Geometry check sheet. Reference: the model listing, model coordinates, mm. A direction names the side the tool comes from. Round coordinates to 2 decimals unless told otherwise and drop trailing zeros. Loops run counter-clockwise (first coordinate to the right, second up) from the corner with the lowest first, then second, coordinate; pieces in that order, holes last.
```python
from build123d import *

# Parameters (mm, degrees)
SKETCH1_R           = 6.35
BOSS_EXTRUDE1_DEPTH = 44.45
CUT_EXTRUDE1_DEPTH  = 129.116424162
FILLET1_R           = 15.9004


with BuildPart() as part:
    # Sketch1 → Boss-Extrude1 (new, symmetric)
    with BuildSketch(Plane.XY):
        with BuildLine():
            Line((-35.56, 0), (-35.56, -96.8502))
            Line((-35.56, -96.8502), (35.56, -96.8502))
            Line((35.56, -96.8502), (35.56, 0))
            ThreePointArc((35.56, 0), (0, 35.56), (-35.56, 0))
        make_face()
        Circle(SKETCH1_R, mode=Mode.SUBTRACT)
    extrude(amount=BOSS_EXTRUDE1_DEPTH, both=True)

    # Sketch2 → Cut-Extrude1 (cut, through all)
    with BuildSketch(Plane(origin=(35.56, 0, 0), x_dir=(0, 0, -1), z_dir=(1, 0, 0))):
        with BuildLine():
            Line((-36.4998, 50.8), (36.4998, 50.8))
            Line((36.4998, 50.8), (36.4998, -80.9498))
            ThreePointArc((36.4998, -80.9498), (34.171240332, -86.571440332), (28.5496, -88.9))
            Line((28.5496, -88.9), (-28.5496, -88.9))
            ThreePointArc((-28.5496, -88.9), (-34.171240332, -86.571440332), (-36.4998, -80.9498))
            Line((-36.4998, -80.9498), (-36.4998, 50.8))
        make_face()
    extrude(amount=-CUT_EXTRUDE1_DEPTH, mode=Mode.SUBTRACT)

    # Fillet1
    fillet1_edges = [part.edges().sort_by_distance(p)[0] for p in [
        (0, -96.8502, 44.45),
        (0, -96.8502, -44.45),
    ]]
    fillet(fillet1_edges, radius=FILLET1_R)


solid = part.part
```
1) Sectioned sample at C-C, the plane x = 21. Record the cut outline in (y, z).
Report:
outline: (-96.85, -28.55) arc R15.9 ccw to (-80.95, -44.45) - (28.7, -44.45) - (28.7, -36.5) - (-80.95, -36.5) arc R7.95 cw to (-88.9, -28.55) - (-88.9, 28.55) arc R7.95 cw to (-80.95, 36.5) - (28.7, 36.5) - (28.7, 44.45) - (-80.95, 44.45) arc R15.9 ccw to (-96.85, 28.55) - close
2) Sectioned sample at A-A, the plane x = 0. Record the cut outline in (y, z), then the cut area to 3 significant figures.
Report:
outline: (-96.85, -28.55) arc R15.9 ccw to (-80.95, -44.45) - (-6.35, -44.45) - (-6.35, -36.5) - (-80.95, -36.5) arc R7.95 cw to (-88.9, -28.55) - (-88.9, 28.55) arc R7.95 cw to (-80.95, 36.5) - (-6.35, 36.5) - (-6.35, 44.45) - (-80.95, 44.45) arc R15.9 ccw to (-96.85, 28.55) - close; (6.35, -44.45) - (35.56, -44.45) - (35.56, -36.5) - (6.35, -36.5) - close; (6.35, 36.5) - (35.56, 36.5) - (35.56, 44.45) - (6.35, 44.45) - close
area: 2,400 mm2
3) Gauge pin test, flat end, axial feed: pin 1 (1 mm diameter, centred on x = -2, y = -82.5, fed in from -Z). Record the tip position at first contact, or that the pin passes through.
Report:
pin 1: stops at z = -44.42
4) Scan lines: line 1 along X through (y, z) = (0, -38.25); line 2 along Z through (x, y) = (-28, -53.5); line 3 along Y through (x, z) = (-23.5, 14.5). Record each from-to range of solid material in increasing order.
Report:
line 1: x = -35.56 to -6.35, 6.35 to 35.56
line 2: z = -44.45 to -36.5, 36.5 to 44.45
line 3: y = -96.85 to -88.9
5) Mould release check, pull along X, two halves, no side actions. Record for faces 1 (the face through (0.78, 35.55, 40.53)), 2 (the face through (-1.38, -6.2, 40.42)), 3 (the face through (0, -22, -44.45)): +X half, -X half, draft (parallel to the pull), parting line (faces both ways), or undercut.
Report:
face 1: parting line
face 2: undercut
face 3: draft
6) Sectioned sample at D-D, the plane z = 5. Record the cut outline in (x, y).
Report:
outline: (-35.56, -96.85) - (35.56, -96.85) - (35.56, -88.9) - (-35.56, -88.9) - close
7) Access from +Z, -Z, +X, -X, +Y, -Y to the whole of each face (thin tool, end or side, straight path). Record for faces 4 (the face through (0.78, 35.55, -40.42)), 5 (the face through (0.5, -86.51, -34.23)).
Report:
face 4: +Z, -Z, +Y
face 5: +X, -X, +Y
8) Sectioned sample at B-B, the plane y = -54.5. Record the cut outline in (x, z), then the cut area to 3 significant figures.
Report:
outline: (-35.56, -44.45) - (35.56, -44.45) - (35.56, -36.5) - (-35.56, -36.5) - close; (-35.56, 36.5) - (35.56, 36.5) - (35.56, 44.45) - (-35.56, 44.45) - close
area: 1,130 mm2
